Read the model definition and answer for the solid it produces. Units are mm, in the model's axes. Round coordinates to 2 decimals unless told otherwise and drop trailing zeros. Write each loop counter-clockwise with the first axis right and the second up, starting at its lowest first coordinate (ties: lowest second). Pieces come first, ordered by that corner, then holes. Notation, with made-up numbers: (68, 87.5) - (76, 87.5) arc R21 cw to (76, 99.5) - close; hole circle Ø10 at (21, 15.5). An arc over 180 degrees is marked (long way). Use one line per item in the form item = value. Start each with the question number.
1) The part is cut by section C-C, the plane z = 33. Give the vertices of the cut face in (x, y), plus the area to 3 significant figures.
2) For a pull along X with two mould halves and no side action, classify faces 1 (the face through (27.46, 1.48, 9.83)), 2 (the face through (9.667, 1.479, -1.269)), 3 (the face through (-1, 1, 40)) as released by +X, released by -X, zero draft, split by the parting line, or undercut.
3) Consider line 1 along X through (y, z) = (1.7, 33); line 2 along Z through (x, y) = (0.5, 1.6); line 3 along X through (y, z) = (2.1, 35). Determine where each line is inside the solid, lowest interval first. Write a range as from..to.
4) The part is cut by section D-D, the plane z = 5. Give the vertices of the cut face in (x, y), plus the area to 3 significant figures.
5) Each of these flat-tipped pins is pushed along its axis until it touches: pin 1 (10 mm diameter, centred on x = 0, z = 1, fed in from +Y); pin 2 (1.5 mm diameter, centred on y = 1.5, z = -3.5, fed in from -X). Where does it stop, or does it pass through?
6) The part is cut by section A-A, the plane x = 0. Give the vertices of the cut face in (y, z).
7) The part is cut by section B-B, the plane y = 1.15. Give the vertices of the cut face in (x, z).
from build123d import *

# Parameters (mm, degrees)
SKETCH1_R            = 9.75
BOSS_EXTRUDE1_DEPTH  = 3
M5_CLEARANCE_HOLE1_D = 5.3


with BuildPart() as part:
    # Sketch1 → Boss-Extrude1 (new body)
    with BuildSketch(Plane(origin=(0, 0, 0), x_dir=(1, 0, 0), z_dir=(0, 1, 0))):
        with BuildLine():
            Line((-9.377695636, 9.003267438), (-45.049528419, -28.152086764))
            ThreePointArc((-45.049528419, -28.152086764), (-46.439541624, -35.744504268), (-40, -40))
            Line((-40, -40), (40, -40))
            ThreePointArc((40, -40), (46.439541624, -35.744504268), (45.049528419, -28.152086764))
            Line((45.049528419, -28.152086764), (9.377695636, 9.003267438))
            ThreePointArc((9.377695636, 9.003267438), (0, 13), (-9.377695636, 9.003267438))
        make_face()
        with Locations(Location((0, 0, 0), (0, 0, 270))):
            Circle(SKETCH1_R, mode=Mode.SUBTRACT)
    extrude(amount=BOSS_EXTRUDE1_DEPTH)

    # M5 Clearance Hole1 (through all)
    with Locations(Plane(origin=(0, 3, 0), x_dir=(1, 0, 0), z_dir=(0, 1, 0))):
        with Locations((-40, -33), (40, -33)):
            Hole(M5_CLEARANCE_HOLE1_D / 2)


solid = part.part
Geometry results:
q1.outline = (-47, 0) - (-42.65, 0) - (-42.65, 3) - (-47, 3) - close; (-37.35, 0) - (37.35, 0) - (37.35, 3) - (-37.35, 3) - close; (42.65, 0) - (47, 0) - (47, 3) - (42.65, 3) - close
q1.area = 250 mm2
q2.face_1 = released by +X
q2.face_2 = undercut
q2.face_3 = zero draft
q3.line_1 = -47..-42.65, -37.35..37.35, 42.65..47
q3.line_2 = -12.99..-9.74, 9.74..40
q3.line_3 = -46.71..-41.74, -38.26..38.26, 41.74..46.71
q4.outline = (-22.82, 0) - (-8.37, 0) - (-8.37, 3) - (-22.82, 3) - close; (8.37, 0) - (22.82, 0) - (22.82, 3) - (8.37, 3) - close
q4.area = 86.7 mm2
q5.pin_1 = through
q5.pin_2 = -15.38
q6.outline = (0, -13) - (3, -13) - (3, -9.75) - (0, -9.75) - close; (0, 9.75) - (3, 9.75) - (3, 40) - (0, 40) - close
q7.outline = (-45.05, 28.15) - (-9.38, -9) arc R13 ccw to (9.38, -9) - (45.05, 28.15) arc R7 ccw to (40, 40) - (-40, 40) arc R7 ccw to start; hole circle Ø5.3 at (-40, 33); hole circle Ø19.5 at (0, 0); hole circle Ø5.3 at (40, 33)
